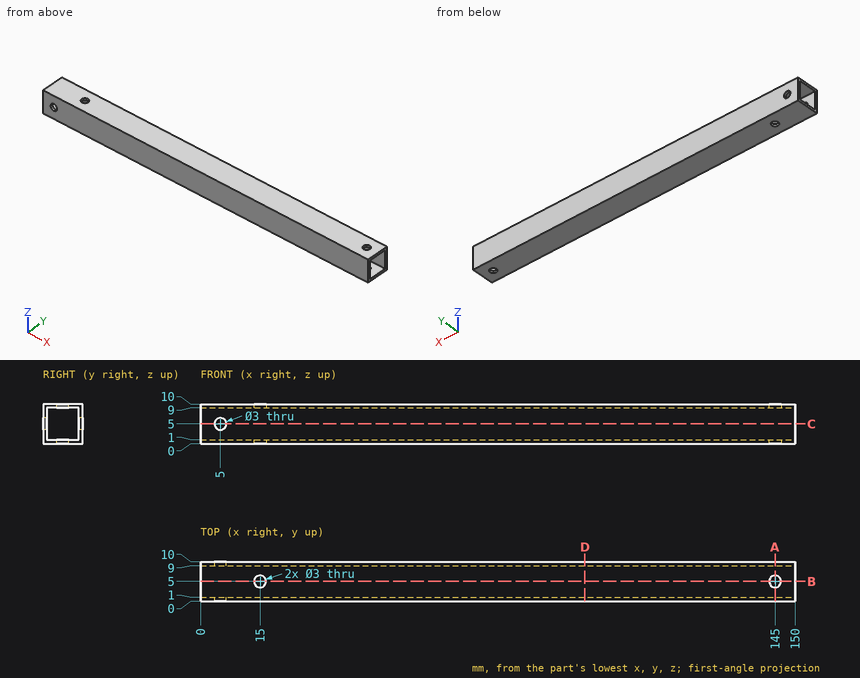
For this review, use the dimensioned drawing (mm, ordinates from the lowest corner) and the shaded views. Round coordinates to 2 decimals unless told otherwise and drop trailing zeros. Order: outer loops, then holes, each group sorted by start corner. A loop starts at its lowest first (then second) coordinate and runs counter-clockwise, first axis right, second up. Notation, with made-up numbers: M 0,87.25 L 36,87.25 A25 cw 36,123.25 Z; hole C 42.5,-4.5 d6. An arc over 180 degrees is marked long. Use a Markdown table: item, result.
1) Insertion check: pin 1 (1.8 mm diameter, centred on x = 145, y = 5, fed in from -Z). The pin has a flat end and moves straight along its axis. Give the tip position at first contact, or say it passes through.
Report:
| item | result |
|---|---|
| pin 1 | through |
2) Consider section D-D (x = 97). Write out the cut boundary in (y, z), then the cut area to 3 significant figures.
Report:
| item | result |
|---|---|
| outline | M 0,0 L 10,0 L 10,10 L 0,10 Z; hole M 1,1 L 9,1 L 9,9 L 1,9 Z |
| area | 36.0 mm^2 |
3) Consider section A-A (x = 145). Write out the cut boundary in (y, z), then the cut area to 3 significant figures.
Report:
| item | result |
|---|---|
| outline | M 0,0 L 3.5,0 L 3.5,1 L 1,1 L 1,9 L 3.5,9 L 3.5,10 L 0,10 Z; M 6.5,0 L 10,0 L 10,10 L 6.5,10 L 6.5,9 L 9,9 L 9,1 L 6.5,1 Z |
| area | 30.0 mm^2 |
4) Consider section C-C (z = 5). Write out the cut boundary in (x, y), then the cut area to 3 significant figures.
Report:
| item | result |
|---|---|
| outline | M 0,0 L 3.5,0 L 3.5,1 L 0,1 Z; M 0,9 L 3.5,9 L 3.5,10 L 0,10 Z; M 6.5,0 L 150,0 L 150,1 L 6.5,1 Z; M 6.5,9 L 150,9 L 150,10 L 6.5,10 Z |
| area | 294 mm^2 |
5) Consider section B-B (y = 5). Write out the cut boundary in (x, z), then the cut area to 3 significant figures.
Report:
| item | result |
|---|---|
| outline | M 0,0 L 13.5,0 L 13.5,1 L 0,1 Z; M 0,9 L 13.5,9 L 13.5,10 L 0,10 Z; M 16.5,0 L 143.5,0 L 143.5,1 L 16.5,1 Z; M 16.5,9 L 143.5,9 L 143.5,10 L 16.5,10 Z; M 146.5,0 L 150,0 L 150,1 L 146.5,1 Z; M 146.5,9 L 150,9 L 150,10 L 146.5,10 Z |
| area | 288 mm^2 |
6) Wall thickness on line 1 along Y through (x, z) = (91, 2.5); line 2 along Z through (x, y) = (5, 9.7): over which ranges is each line inside the solid? List them lowest first. Write a range as [from, to].
Report:
| item | result |
|---|---|
| line 1 | [0, 1], [9, 10] |
| line 2 | [0, 3.5], [6.5, 10] |
